Read the model definition and answer for the solid it produces. Units are mm, in the model's axes. Give positions to 0.01 mm unless a question says otherwise; leave off trailing zeros. Order: outer loops, then holes, each group sorted by start corner. A loop starts at its lowest first (then second) coordinate and runs counter-clockwise, first axis right, second up. Notation, with made-up numbers: (49, 62) - (54, 62) arc R23 ccw to (54, 77) - close; hole circle Ø9 at (10, -10.75). An arc over 180 degrees is marked (long way). Return JSON: item names as keys, results as strings.
```python
from build123d import *

# Parameters (mm, degrees)
SKETCH_2_W          = 220
SKETCH_2_H          = 220
SKETCH_2_W_2        = 35
SKETCH_2_H_2        = 80
SKETCH_2_W_3        = 70
SKETCH_2_H_3        = 20
EXTRUDE_1_DEPTH     = 2
SKETCH_3_R          = 2
CUT_EXTRUDE_1_DEPTH = 2


with BuildPart() as part:
    # Эскиз2 → Бобышка-Вытянуть1 (new body)
    with BuildSketch(Plane(origin=(0, 0, 0), x_dir=(1, 0, 0), z_dir=(0, 1, 0))):
        with Locations((110, 110)):
            Rectangle(SKETCH_2_W, SKETCH_2_H)
        with Locations((27.5, 170)):
            Rectangle(SKETCH_2_W_2, SKETCH_2_H_2, mode=Mode.SUBTRACT)
        with Locations((110, 170)):
            Rectangle(SKETCH_2_W_3, SKETCH_2_H_2, mode=Mode.SUBTRACT)
        with Locations((192.5, 170)):
            Rectangle(SKETCH_2_W_2, SKETCH_2_H_2, mode=Mode.SUBTRACT)
        with Locations((192.5, 50)):
            Rectangle(SKETCH_2_W_2, SKETCH_2_H_2, mode=Mode.SUBTRACT)
        with Locations((110, 50)):
            Rectangle(SKETCH_2_W_3, SKETCH_2_H_2, mode=Mode.SUBTRACT)
        with Locations((27.5, 50)):
            Rectangle(SKETCH_2_W_2, SKETCH_2_H_2, mode=Mode.SUBTRACT)
        with Locations((27.5, 110)):
            Rectangle(SKETCH_2_W_2, SKETCH_2_H_3, mode=Mode.SUBTRACT)
        with Locations((192.5, 110)):
            Rectangle(SKETCH_2_W_2, SKETCH_2_H_3, mode=Mode.SUBTRACT)
    extrude(amount=EXTRUDE_1_DEPTH)

    # Эскиз3 → Вырез-Вытянуть1 (cut)
    with BuildSketch(Plane(origin=(0, 2, 0), x_dir=(1, 0, 0), z_dir=(0, 1, 0))):
        with Locations(Location((171.5, 26.5, 0), (0, 0, 270))):
            Circle(SKETCH_3_R)
        with Locations(Location((148.5, 26.5, 0), (0, 0, 270))):
            Circle(SKETCH_3_R)
        with Locations(Location((71.5, 26.5, 0), (0, 0, 270))):
            Circle(SKETCH_3_R)
        with Locations(Location((48.5, 26.5, 0), (0, 0, 270))):
            Circle(SKETCH_3_R)
        with Locations(Location((48.5, 63.5, 0), (0, 0, 270))):
            Circle(SKETCH_3_R)
        with Locations(Location((71.5, 63.5, 0), (0, 0, 270))):
            Circle(SKETCH_3_R)
        with Locations(Location((148.5, 63.5, 0), (0, 0, 270))):
            Circle(SKETCH_3_R)
        with Locations(Location((171.5, 63.5, 0), (0, 0, 270))):
            Circle(SKETCH_3_R)
        with Locations(Location((171.5, 156.5, 0), (0, 0, 270))):
            Circle(SKETCH_3_R)
        with Locations(Location((148.5, 156.5, 0), (0, 0, 270))):
            Circle(SKETCH_3_R)
        with Locations(Location((148.5, 193.5, 0), (0, 0, 270))):
            Circle(SKETCH_3_R)
        with Locations(Location((171.5, 193.5, 0), (0, 0, 270))):
            Circle(SKETCH_3_R)
        with Locations(Location((71.5, 193.5, 0), (0, 0, 270))):
            Circle(SKETCH_3_R)
        with Locations(Location((71.5, 156.5, 0), (0, 0, 270))):
            Circle(SKETCH_3_R)
        with Locations(Location((48.5, 156.5, 0), (0, 0, 270))):
            Circle(SKETCH_3_R)
        with Locations(Location((48.5, 193.5, 0), (0, 0, 270))):
            Circle(SKETCH_3_R)
    extrude(amount=-CUT_EXTRUDE_1_DEPTH, mode=Mode.SUBTRACT)


solid = part.part
```
Q1. A cutting plane is placed at C-C (z = -43.5). Write down the section's boundary in (x, y), and give its area (3 significant figures).
Values:
{"outline": "(0, 0) - (10, 0) - (10, 2) - (0, 2) - close; (45, 0) - (75, 0) - (75, 2) - (45, 2) - close; (145, 0) - (175, 0) - (175, 2) - (145, 2) - close; (210, 0) - (220, 0) - (220, 2) - (210, 2) - close", "area": "160 mm²"}
Q2. A cutting plane is placed at A-A (x = 137.5). Write down the section's boundary in (y, z).
Values:
{"outline": "(0, -220) - (2, -220) - (2, -210) - (0, -210) - close; (0, -130) - (2, -130) - (2, -90) - (0, -90) - close; (0, -10) - (2, -10) - (2, 0) - (0, 0) - close"}
Q3. A cutting plane is placed at B-B (x = 29). Write down the section's boundary in (y, z).
Values:
{"outline": "(0, -220) - (2, -220) - (2, -210) - (0, -210) - close; (0, -130) - (2, -130) - (2, -120) - (0, -120) - close; (0, -100) - (2, -100) - (2, -90) - (0, -90) - close; (0, -10) - (2, -10) - (2, 0) - (0, 0) - close"}
Q4. Consider L1, parallel to X at y = 1.1, z = -208; L2, parallel to Z at x = 148.5, y = 0.45; L3, parallel to Z at x = 90, y = 1.5. Determine where each line is inside the solid, lowest interval first.
Values:
{"L1": "x = 0 to 10, 45 to 75, 145 to 175, 210 to 220", "L2": "z = -220 to -195.5, -191.5 to -158.5, -154.5 to -65.5, -61.5 to -28.5, -24.5 to 0", "L3": "z = -220 to -210, -130 to -90, -10 to 0"}
Q5. A cutting plane is placed at D-D (y = 0.75). Give the number of separate pieces and of enclosed holes in the cut face, and give its area (3 significant figures).
Values:
{"separate pieces": "1", "enclosed holes": "24", "area": "24,400 mm²"}
